from build123d import *

# Parameters (mm, degrees)
SKETCH1_W           = 60
SKETCH1_H           = 60
SKETCH1_W_2         = 50
SKETCH1_H_2         = 50
BOSS_EXTRUDE1_DEPTH = 60
SKETCH2_W           = 60
SKETCH2_H           = 60
BOSS_EXTRUDE2_DEPTH = 5
SKETCH3_R           = 1.25
CUT_EXTRUDE1_DEPTH  = 5
CUT_EXTRUDE2_REACH  = 62
SKETCH4_R           = 1.25
CHAMFER1_SIZE       = 10
CUT_EXTRUDE4_REACH  = 62
SKETCH6_W           = 2
SKETCH6_H           = 2


with BuildPart() as part:
    # Sketch1 → Boss-Extrude1 (new body)
    with BuildSketch(Plane(origin=(0, 0, 0), x_dir=(1, 0, 0), z_dir=(0, 1, 0))):
        Rectangle(SKETCH1_W, SKETCH1_H)
        Rectangle(SKETCH1_W_2, SKETCH1_H_2, mode=Mode.SUBTRACT)
    extrude(amount=BOSS_EXTRUDE1_DEPTH)

    # Sketch2 → Boss-Extrude2 (add)
    with BuildSketch(Plane.XZ):
        Rectangle(SKETCH2_W, SKETCH2_H)
    extrude(amount=BOSS_EXTRUDE2_DEPTH)

    # Sketch3 → Cut-Extrude1 (cut)
    with BuildSketch(Plane(origin=(0, 0, -30), x_dir=(-1, 0, 0), z_dir=(0, 0, -1))):
        with Locations((0, 2.5)):
            Circle(SKETCH3_R)
        with Locations((0, 8.1)):
            Circle(SKETCH3_R)
    extrude(amount=-CUT_EXTRUDE1_DEPTH, mode=Mode.SUBTRACT)

    # Sketch4 → Cut-Extrude2 (cut, up to next)
    with BuildSketch(Plane(origin=(0, 0, -30), x_dir=(-1, 0, 0), z_dir=(0, 0, -1)), mode=Mode.PRIVATE) as cut_extrude2_sk1:
        with Locations((-13.176528006, 8.1)):
            Circle(SKETCH4_R)
    cut_extrude2_tool1 = extrude(cut_extrude2_sk1.sketch, amount=-CUT_EXTRUDE2_REACH, mode=Mode.PRIVATE) & part.part
    add(cut_extrude2_tool1.solids().sort_by_distance((13.176528, 8.1, -30))[0], mode=Mode.SUBTRACT)

    # Chamfer1
    chamfer1_edges = [part.edges().sort_by_distance(p)[0] for p in [
        (25, 30, 25),
        (25, 30, -25),
        (-25, 30, -25),
        (-25, 30, 25),
    ]]
    chamfer(chamfer1_edges, length=CHAMFER1_SIZE)

    # Sketch6 → Cut-Extrude4 (cut, up to next)
    with BuildSketch(Plane.XY.offset(30), mode=Mode.PRIVATE) as cut_extrude4_sk1:
        with Locations((0, 1)):
            Rectangle(SKETCH6_W, SKETCH6_H)
    cut_extrude4_tool1 = extrude(cut_extrude4_sk1.sketch, amount=-CUT_EXTRUDE4_REACH, mode=Mode.PRIVATE) & part.part
    add(cut_extrude4_tool1.solids().sort_by_distance((0, 1, 30))[0], mode=Mode.SUBTRACT)


solid = part.part
Model file for the job. Use its own axes, mm. A direction names the side the tool comes from. Give positions to 0.01 mm unless a question says otherwise; leave off trailing zeros. Loops run counter-clockwise (first coordinate to the right, second up) from the corner with the lowest first, then second, coordinate; pieces in that order, holes last.
1) Saw through at C-C (x = -20). Write the cut outline in (y, z), plus the area to 3 significant figures.
2) Saw through at B-B (y = 8.1). Write the cut outline in (x, z).
3) Wall check: line 1 (Y direction, x = 0, z = -28.5); line 2 (X direction, y = 8, z = -27); line 3 (Z direction, x = 11.5, y = 52). Give the ranges that are in metal, low to high.
4) Flat gauge pin, fed straight in: pin 1 Ø2 at (x, z) = (-8.5, -10.5) entering from +Y. Where does the tip first touch, or does it go through?
5) Tool access for faces 1 (the flat face through (1, 1, 28)), 2 (the flat face through (-20, 30, -20)), 3 (the cylindrical face through (12.022, 7.621, -27.535)): list every direction of +Z, -Z, +X, -X, +Y, -Y with a clear straight run to the whole face (end or side of a thin tool).
6) Saw through at D-D (y = 25.5). Write the cut outline in (x, z), plus the area to 3 significant figures.
7) Pull direction Y, two halves, no side cores. Call faces 4 (the cylindrical face through (0.16, 3.74, -27.54)), 5 (the flat face through (-20, 30, 20)), 6 (the flat face through (0, -5, 0)): +Y half, -Y half, draft (parallel to the pull), parting line (faces both ways), or undercut.
8) Saw through at A-A (x = 0). Write the cut outline in (y, z), plus the area to 3 significant figures.
Answer block:
1. outline: (-5, -30) - (60, -30) - (60, -20) - (0, -20) - (0, 20) - (60, 20) - (60, 30) - (-5, 30) - close
1. area: 1,500 mm2
2. outline: (-30, -30) - (-1.25, -30) - (-1.25, -25) - (-15, -25) - (-25, -15) - (-25, 15) - (-15, 25) - (15, 25) - (25, 15) - (25, -15) - (15, -25) - (14.43, -25) - (14.43, -30) - (30, -30) - (30, 30) - (-30, 30) - close; (1.25, -30) - (11.93, -30) - (11.93, -25) - (1.25, -25) - close
3. line 1: y = -5 to 1.25, 3.75 to 6.85, 9.35 to 60
3. line 2: x = -30 to -1.25, 1.25 to 11.93, 14.42 to 30
3. line 3: z = -30 to -25, 25 to 30
4. pin 1: stops at y = 0
5. face 1: +Z
5. face 2: +Y
5. face 3: -Z
6. outline: (-30, -30) - (30, -30) - (30, 30) - (-30, 30) - close; hole (-25, -15) - (-15, -25) - (15, -25) - (25, -15) - (25, 15) - (15, 25) - (-15, 25) - (-25, 15) - close
6. area: 1,300 mm2
7. face 4: undercut
7. face 5: draft
7. face 6: -Y half
8. outline: (-5, -30) - (1.25, -30) - (1.25, -25) - (0, -25) - (0, 30) - (-5, 30) - close; (2, 25) - (60, 25) - (60, 30) - (2, 30) - close; (3.75, -30) - (6.85, -30) - (6.85, -25) - (3.75, -25) - close; (9.35, -30) - (60, -30) - (60, -25) - (9.35, -25) - close
8. area: 865 mm2
